For this review, take the finished solid that the model builds, in its own axes (mm). A direction names the side the tool comes from. Give positions to 0.01 mm unless a question says otherwise; leave off trailing zeros. Order: outer loops, then holes, each group sorted by start corner. A loop starts at its lowest first (then second) coordinate and runs counter-clockwise, first axis right, second up. Notation, with made-up numbers: (50.5, -16) - (54.5, -16) arc R20 ccw to (54.5, 0) - close; hole circle Ø2 at (61, -11.75). An arc over 180 degrees is marked (long way). Answer as a JSON object with one key per item and string values. Group by question number.
from build123d import *

# Parameters (mm, degrees)
F1_DEPTH = 88.9


with BuildPart() as f1:
    # F0 (on Right) → F1 (new body)
    with BuildSketch(Plane.YZ):
        with BuildLine():
            ThreePointArc((-32.662655, 15.440298), (-38.465343, 23.557587), (-38.769789, 33.530996))
            ThreePointArc((-38.769789, 33.530996), (-47.167676, 17.086921), (-36.802551, 1.806337))
            ThreePointArc((-36.802551, 1.806337), (-34.138246, 1.199843), (-31.465744, 1.769124))
            Line((-31.465744, 1.769124), (80.485985, 52.669767))
            Line((80.485985, 52.669767), (-26.662719, 14.49403))
            ThreePointArc((-26.662719, 14.49403), (-29.783168, 14.20324), (-32.662655, 15.440298))
        make_face()
    extrude(amount=F1_DEPTH)


solid = f1.part
1) Consider section A-A (z = 21). Give the boundary of the cut face in (x, y), plus the area to 3 significant figures.
2) For faces 5 (the face through (43.83, 27.66, 33.85)), 6 (the face through (0, -12, 19)), list the 3-axis set-ups (+Z, -Z, +X, -X, +Y, -Y) from which the entire face can be reached by the end or side of a thin tool; tool diameter is ignored.
3) Consider section B-B (x = 48.5). Give the boundary of the cut face in (y, z), plus the area to 3 significant figures.
4) Mouldability with a two-part tool opening along Y and no side actions: class faces 1 (the face through (43.8, -34.2, 1.2)), 2 (the face through (43.828, -47.182, 17.358)), 3 (the face through (43.83, -38.42, 23.42)), 4 (the face through (43.828, -29.739, 14.196)) as released by +Y, released by -Y, zero draft, split by the parting line, or undercut.
5) For pin 1 (4 mm diameter, centred on x = 65.5, y = -19, fed in from -Z); pin 2 (5 mm diameter, centred on x = 20, z = 31, fed in from +Y); pin 3 (2 mm diameter, centred on x = 52.5, y = -23.5, fed in from +Z), all flat-tipped, find the tip position at first contact; note any pin that passes through.
6) Consider section D-D (z = 40). Give the boundary of the cut face in (x, y).
7) For line 1 (Z direction, x = 67.5, y = 24.5); line 2 (Z direction, x = 76.5, y = -41); line 3 (Y direction, x = 64, z = 8), list the stretches that pass through material, from the lowest coordinate up.
8) Consider section C-C (y = 42). Give the boundary of the cut face in (x, z).
Result set:
{
 "1": {"outline": "(0, -46.99) - (88.9, -46.99) - (88.9, -37.36) - (0, -37.36) - close; (0, -8.4) - (88.9, -8.4) - (88.9, 10.83) - (0, 10.83) - close", "area": "2,570 mm2"},
 "2": {"face 5": "+Z, +X, -X", "face 6": "+Z, -Z, -X, +Y, -Y"},
 "3": {"outline": "(-38.77, 33.53) arc R18.14 ccw to (-36.8, 1.81) arc R6.35 ccw to (-31.47, 1.77) - (80.49, 52.67) - (-26.66, 14.49) arc R6.35 cw to (-32.66, 15.44) arc R17.16 cw to start", "area": "920 mm2"},
 "4": {"face 1": "split by the parting line", "face 2": "released by -Y", "face 3": "undercut", "face 4": "undercut"},
 "5": {"pin 1": "stops at z = 6.53", "pin 2": "stops at y = 38.32", "pin 3": "stops at z = 15.98"},
 "6": {"outline": "(0, 44.93) - (88.9, 44.93) - (88.9, 52.62) - (0, 52.62) - close"},
 "7": {"line 1": "z = 27.21 to 32.72", "line 2": "z = 4.55 to 31.87", "line 3": "y = -44.06 to -17.76"},
 "8": {"outline": "(0, 35.17) - (88.9, 35.17) - (88.9, 38.96) - (0, 38.96) - close"}
}
